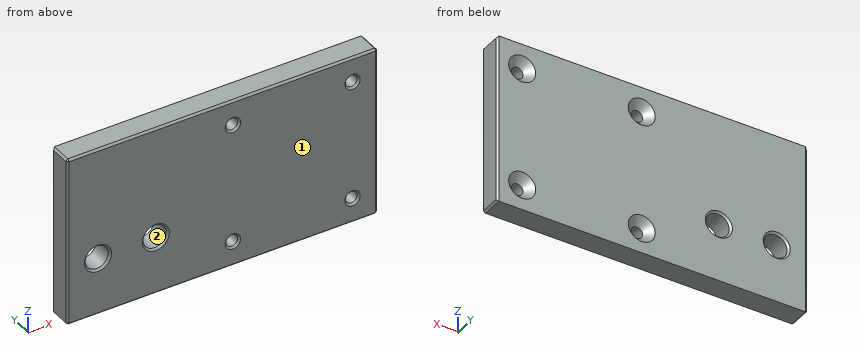
from build123d import *

# Parameters (mm, degrees)
CROQUIS1_W              = 80.5
CROQUIS1_H              = 44
CROQUIS1_R              = 1.5
CROQUIS1_R_2            = 3
SALIENTE_EXTRUIR1_DEPTH = 6
CHAFL_N1_SIZE           = 0.5
CHAFL_N2_SIZE           = 2


with BuildPart() as part:
    # Croquis1 → Saliente-Extruir1 (new body)
    with BuildSketch(Plane(origin=(0, 0, 0), x_dir=(1, 0, 0), z_dir=(0, 1, 0))):
        with Locations((7.521686308, -1.221461187)):
            Rectangle(CROQUIS1_W, CROQUIS1_H)
        with Locations(Location((10.271686308, 14.278538813, 0), (0, 0, 270))):
            Circle(CROQUIS1_R, mode=Mode.SUBTRACT)
        with Locations(Location((41.271686308, 14.278538813, 0), (0, 0, 270))):
            Circle(CROQUIS1_R, mode=Mode.SUBTRACT)
        with Locations(Location((10.271686308, -16.721461187, 0), (0, 0, 270))):
            Circle(CROQUIS1_R, mode=Mode.SUBTRACT)
        with Locations(Location((41.271686308, -16.721461187, 0), (0, 0, 270))):
            Circle(CROQUIS1_R, mode=Mode.SUBTRACT)
        with Locations(Location((-24.728313692, 5.778538813, 0), (0, 0, 270))):
            Circle(CROQUIS1_R_2, mode=Mode.SUBTRACT)
        with Locations(Location((-9.728313692, 5.778538813, 0), (0, 0, 270))):
            Circle(CROQUIS1_R_2, mode=Mode.SUBTRACT)
    extrude(amount=SALIENTE_EXTRUIR1_DEPTH)

    # Chaflán1
    chafl_n1_edges = [part.edges().sort_by_distance(p)[0] for p in [
        (47.771686308, 6, 1.221461187),
        (10.271686308, 0, -15.778538813),
        (41.271686308, 0, -15.778538813),
        (10.271686308, 0, 15.221461187),
        (41.271686308, 0, 15.221461187),
        (-24.728313692, 0, -8.778538813),
        (-24.728313692, 6, -8.778538813),
        (-9.728313692, 0, -8.778538813),
        (-9.728313692, 6, -8.778538813),
        (-32.728313692, 6, 1.221461187),
        (7.521686308, 0, -20.778538813),
        (47.771686308, 0, 1.221461187),
        (7.521686308, 0, 23.221461187),
        (-32.728313692, 0, 1.221461187),
        (-32.728313692, 3, -20.778538813),
        (47.771686308, 3, -20.778538813),
        (47.771686308, 3, 23.221461187),
        (-32.728313692, 3, 23.221461187),
    ]]
    chamfer(chafl_n1_edges, length=CHAFL_N1_SIZE)

    # Chaflán2
    chafl_n2_edges = [part.edges().sort_by_distance(p)[0] for p in [
        (10.271686308, 6, -15.778538813),
        (41.271686308, 6, -15.778538813),
        (10.271686308, 6, 15.221461187),
        (41.271686308, 6, 15.221461187),
    ]]
    chamfer(chafl_n2_edges, length=CHAFL_N2_SIZE)


solid = part.part
Part model, mm, in its own coordinate system. Face numbers are marked on the shaded views. Give positions to 0.01 mm unless a question says otherwise; leave off trailing zeros. Loops run counter-clockwise (first coordinate to the right, second up) from the corner with the lowest first, then second, coordinate; pieces in that order, holes last. Notation, with made-up numbers: M -10.5,46.5 L 33.5,46.5 A24 cw 33.5,72.5 Z; hole C -29.5,3.25 d11. An arc over 180 degrees is marked long. Put each result on its own line as item: value. Start each with the question number.
1) Probe probe 1 along X at (y, z) = (5, -16.5); probe 2 along X at (y, z) = (1.5, 16); probe 3 along Z at (x, y) = (42.5, 4). List the from-to ranges inside material, lowest first.
2) Flat gauge pins, fed straight in: pin 1 (2.5 mm diameter, centred on x = 10.27, z = 16.72, fed in from -Y); pin 2 (8 mm diameter, centred on x = -24.73, z = -5.78, fed in from +Y). Where does each tip first touch, or does it go through?
3) Saw through at B-B (z = -4). State how many separate pieces and enclosed holes the cut face has, then the cut area to 3 significant figures.
4) Saw through at A-A (y = 3). List the corners of the cut face in (x, z).
5) Pull direction X, two halves, no side cores. Call the marked faces 1 and 2: +X half, -X half, draft (parallel to the pull), parting line (faces both ways), or undercut.
Numbers:
1. probe 1: -32.73 to 9.12, 11.42 to 40.12, 42.42 to 47.77
1. probe 2: -32.73 to 8.96, 11.59 to 39.96, 42.59 to 47.77
1. probe 3: -20.78 to -15.14, -13.42 to 15.86, 17.58 to 23.22
2. pin 1: through
2. pin 2: y = 6
3. separate pieces: 3
3. enclosed holes: 0
3. area: 423 mm^2
4. outline: M -32.73,-20.28 L -32.23,-20.78 L 47.27,-20.78 L 47.77,-20.28 L 47.77,22.72 L 47.27,23.22 L -32.23,23.22 L -32.73,22.72 Z; hole C -24.73,-5.78 d6; hole C -9.73,-5.78 d6; hole C 10.27,-14.28 d3; hole C 10.27,16.72 d3; hole C 41.27,-14.28 d3; hole C 41.27,16.72 d3
5. face 1: draft
5. face 2: undercut
